Here's how the part is built. I have some questions about the finished solid (model axes, mm). A direction names the side the tool comes from. Give positions to 0.01 mm unless a question says otherwise; leave off trailing zeros. Loops run counter-clockwise (first coordinate to the right, second up) from the corner with the lowest first, then second, coordinate; pieces in that order, holes last. Notation, with made-up numbers: (88.5, 10) - (119.5, 10) arc R16 ccw to (119.5, 22) - close; hole circle Ø7 at (9.25, 62.5). An arc over 180 degrees is marked (long way). Use a Markdown table: item, result.
from build123d import *

# Parameters (mm, degrees)
F3_DEPTH      = 51.5
F3_DEPTH_BACK = 51.5
F4_R          = 2.5
F5_T          = -2


with BuildPart() as f3:
    # F2 (on Right) → F3 (new body, two sides)
    with BuildSketch(Plane.YZ) as f3_sk:
        Polygon((-54, 0), (54, 0), (52.6636016283, 25.5), (-52.6636016283, 25.5), align=None)
    extrude(amount=F3_DEPTH)
    extrude(f3_sk.sketch, amount=-F3_DEPTH_BACK)

    # F4
    f4_edges = [f3.edges().sort_by_distance(p)[0] for p in [
        (0, -52.663602, 25.5),
        (-51.5, -53.331801, 12.75),
        (-51.5, 0, 25.5),
        (51.5, 0, 25.5),
        (51.5, -53.331801, 12.75),
        (51.5, 53.331801, 12.75),
        (0, 52.663602, 25.5),
        (-51.5, 53.331801, 12.75),
    ]]
    fillet(f4_edges, radius=F4_R)

    # F5
    f5_openings = [f3.faces().sort_by_distance(p)[0] for p in [
        (0, 0, 0),
    ]]
    offset(amount=F5_T, openings=f5_openings, kind=Kind.INTERSECTION)


solid = f3.part
(1) On a 3-axis mill with a long thin cutter (end or side, diameter ignored), from which of +Z, -Z, +X, -X, +Y, -Y can I reach the whole of each face in a straight line? I mean faces 1 (the face through (49.5, -1, 12)), 2 (the face through (50.79, 52.63, 11.69)). Say none if no direction works.
A:
| item | result |
|---|---|
| face 1 | -Z |
| face 2 | +Z, +X, +Y |
(2) If I drill on line 1 (X direction, y = -32, z = 3.25); line 2 (Z direction, x = -24, y = 40); line 3 (Y direction, x = -10, z = 21.25), over which ranges is the centre line in solid material (lowest first)?
A:
| item | result |
|---|---|
| line 1 | -51.5 to -49.5, 49.5 to 51.5 |
| line 2 | 23.5 to 25.5 |
| line 3 | -52.89 to -50.88, 50.88 to 52.89 |
(3) We'd pull the mould along X, two halves only. Please class faces 3 (the face through (0.686, 53.402, 11.404)), 4 (the face through (51.5, -1, 12)), 5 (the face through (0.7, 51.4, 11.4)): pulls with the +X half, pulls with the -X half, needs draft (parallel to the pull), parting line crosses it, or undercut.
A:
| item | result |
|---|---|
| face 3 | needs draft |
| face 4 | pulls with the +X half |
| face 5 | undercut |
(4) Will these pins go through, and if not, where does the flat tip stop? pin 1 (10 mm diameter, centred on x = 10, z = 4.5, fed in from +Y); pin 2 (4 mm diameter, centred on x = -12, z = 7, fed in from +Y); pin 3 (3 mm diameter, centred on x = -21.5, z = 22.5, fed in from +Y); pin 4 (8 mm diameter, centred on x = 15, z = 9, fed in from -Y).
A:
| item | result |
|---|---|
| pin 1 | y = 54 |
| pin 2 | y = 53.74 |
| pin 3 | y = 52.9 |
| pin 4 | y = -53.74 |
(5) Suppose I cut it at B-B on x = 12.5. Write out the boundary of the cut face in (y, z), plus the area to 3 significant figures.
A:
| item | result |
|---|---|
| outline | (-54, 0) - (-52, 0) - (-50.79, 23.03) arc R0.5 cw to (-50.29, 23.5) - (50.29, 23.5) arc R0.5 cw to (50.79, 23.03) - (52, 0) - (54, 0) - (52.79, 23.13) arc R2.5 ccw to (50.29, 25.5) - (-50.29, 25.5) arc R2.5 ccw to (-52.79, 23.13) - close |
| area | 303 mm2 |
(6) Suppose I cut it at A-A on y = 39.5. Write out the boundary of the cut face in (x, z), plus the area to 3 significant figures.
A:
| item | result |
|---|---|
| outline | (-51.5, 0) - (-49.5, 0) - (-49.5, 23) arc R0.5 cw to (-49, 23.5) - (49, 23.5) arc R0.5 cw to (49.5, 23) - (49.5, 0) - (51.5, 0) - (51.5, 23) arc R2.5 ccw to (49, 25.5) - (-49, 25.5) arc R2.5 ccw to (-51.5, 23) - close |
| area | 297 mm2 |
